Input: dimensioned drawing with shaded views. Units: mm. Origin: part minimum x, y, z. A direction names the side the tool comes from. Round coordinates to 2 decimals unless told otherwise and drop trailing zeros. Order: outer loops, then holes, each group sorted by start corner. A loop starts at its lowest first (then second) coordinate and runs counter-clockwise, first axis right, second up. Notation, with made-up numbers: M 79,15 L 120,15 A21 ccw 120,22 Z; hole C 77.5,42.25 d7. An arc over 180 degrees is marked long. Put each result on its own line as item: value. Start each with the question number.
1) Material intervals for probe 1 along Y at (x, z) = (35, 1.6) (3 decimals); probe 2 along Y at (x, z) = (5, 6); probe 3 along Z at (x, y) = (30.5, 5.5), sorted ascending. Write a range as [from, to].
2) Access query for the marked faces 5, 6 and 7. Directions: +Z, -Z, +X, -X, +Y, -Y. A direction counts if a zero-diameter tool reaches every point of the face in a straight line with its end or side. Return the directions, or none.
3) Section A-A, the plane x = 20. Return loops of the section in (y, z).
4) Section B-B, the plane z = 9.5. Return loops of the section in (x, y).
5) Draft query along Y for the marked faces 1, 2, 3 and 4. Return one class per face: pulls with the +Y half, pulls with the -Y half, needs draft (parallel to the pull), parting line crosses it, or undercut.
6) Section C-C, the plane y = 12. Return loops of the section in (x, z).
7) First-contact query: P1, Ø5.5, axis at x = 35, y = 5, coming from the -Z side; P2, Ø2, axis at y = 19, z = 10, coming from the +X side; P3, Ø5, axis at x = 35, y = 25, coming from the +Z side. Flat tips, straight axial feed; report the tip coordinate or a pass-through.
8) Section D-D, the plane z = 3.5. Return loops of the section in (x, y) (3 decimals), then the cut area to 3 significant figures.
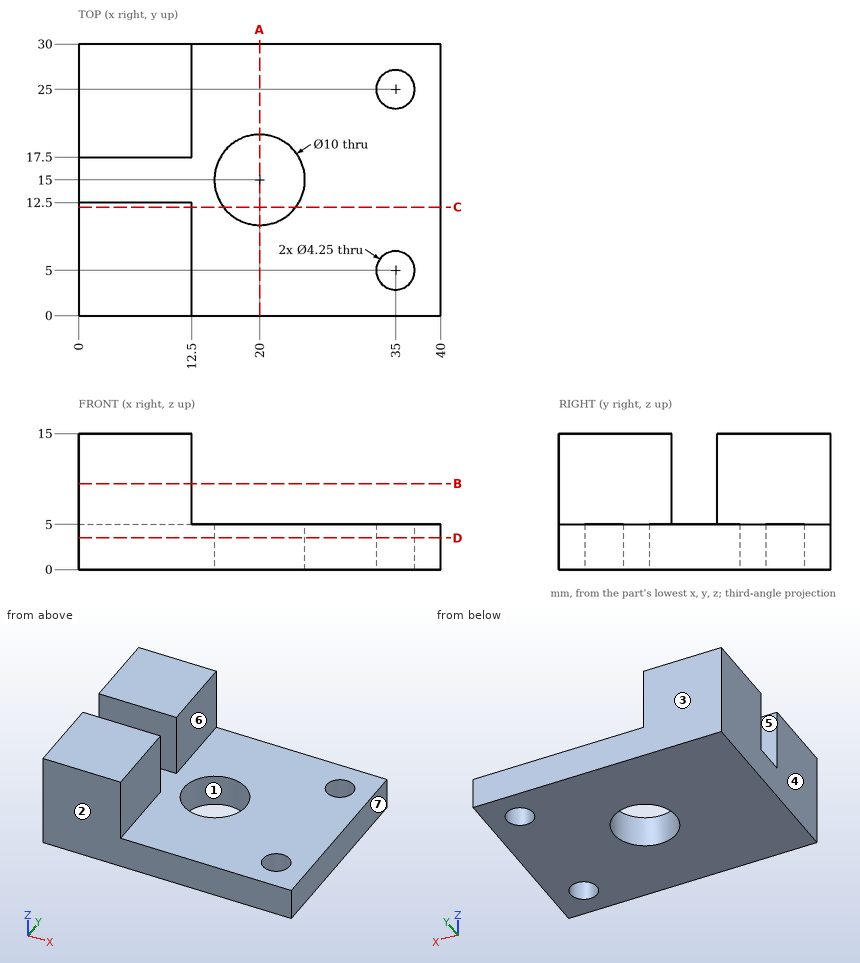
Result sheet:
1. probe 1: y = [0, 2.875], [7.125, 22.875], [27.125, 30]
1. probe 2: y = [0, 12.5], [17.5, 30]
1. probe 3: z = [0, 5]
2. face 5: +Z, +X, -X
2. face 6: +Z, +X, +Y, -Y
2. face 7: +Z, -Z, +X, +Y, -Y
3. outline: M 0,0 L 10,0 L 10,5 L 0,5 Z; M 20,0 L 30,0 L 30,5 L 20,5 Z
4. outline: M 0,0 L 12.5,0 L 12.5,12.5 L 0,12.5 Z; M 0,17.5 L 12.5,17.5 L 12.5,30 L 0,30 Z
5. face 1: undercut
5. face 2: pulls with the -Y half
5. face 3: pulls with the +Y half
5. face 4: needs draft
6. outline: M 0,0 L 16,0 L 16,5 L 12.5,5 L 12.5,15 L 0,15 Z; M 24,0 L 40,0 L 40,5 L 24,5 Z
7. P1: stops at z = 0
7. P2: stops at x = 12.5
7. P3: stops at z = 5
8. outline: M 0,0 L 40,0 L 40,30 L 0,30 Z; hole C 20,15 d10; hole C 35,5 d4.25; hole C 35,25 d4.25
8. area: 1,090 mm2
